```python
from build123d import *

# Parameters (mm, degrees)
BOSS_EXTRUDE1_DEPTH = 7.5
CHAMFER1_SIZE       = 2.5
SKETCH3_W           = 20
SKETCH3_H           = 20
BOSS_EXTRUDE2_DEPTH = 10
CHAMFER4_SIZE       = 2.5
SKETCH6_R           = 5
BOSS_EXTRUDE3_DEPTH = 10
CUT_EXTRUDE3_DEPTH  = 17
SKETCH11_R          = 30
SKETCH11_R_2        = 20
BOSS_EXTRUDE4_DEPTH = 20
CHAMFER5_SIZE2      = 20
CHAMFER5_SIZE       = 5
CHAMFER6_SIZE       = 2.5


with BuildPart() as part:
    # Sketch2 → Boss-Extrude1 (new, symmetric)
    with BuildSketch(Plane.XY):
        with BuildLine():
            ThreePointArc((84.922137279, 7.499595816), (1.268561005, 10.133701432), (-81.871756055, 19.753837344))
            ThreePointArc((-81.871756055, 19.753837344), (-104.803696773, 2.795280684), (-87.461525308, -19.847944306))
            ThreePointArc((-87.461525308, -19.847944306), (0.380210023, -22.09713345), (86.984359422, -7.232725467))
            ThreePointArc((86.984359422, -7.232725467), (92.427584063, 1.039709088), (84.922137279, 7.499595816))
        make_face()
    extrude(amount=BOSS_EXTRUDE1_DEPTH, both=True)

    # Chamfer1
    chamfer1_edges = [part.edges().sort_by_distance(p)[0] for p in [
        (92.427584063, 1.039709088, 7.5),
        (1.268561005, 10.133701432, 7.5),
        (-104.803696773, 2.795280684, 7.5),
        (0.380210023, -22.09713345, 7.5),
        (-104.803696773, 2.795280684, -7.5),
        (1.268561005, 10.133701432, -7.5),
        (92.427584063, 1.039709088, -7.5),
        (0.380210023, -22.09713345, -7.5),
    ]]
    chamfer(chamfer1_edges, length=CHAMFER1_SIZE)

    # Sketch3 → Boss-Extrude2 (add)
    with BuildSketch(Plane.XY.offset(7.5)):
        with Locations((-85, 0)):
            Rectangle(SKETCH3_W, SKETCH3_H)
    extrude(amount=BOSS_EXTRUDE2_DEPTH)

    # Chamfer4
    chamfer4_edges = [part.edges().sort_by_distance(p)[0] for p in [
        (-75, 0, 17.5),
        (-85, 10, 17.5),
        (-95, 0, 17.5),
        (-85, -10, 17.5),
    ]]
    chamfer(chamfer4_edges, length=CHAMFER4_SIZE)

    # Sketch6 → Boss-Extrude3 (add)
    with BuildSketch(Plane(origin=(0, 0, -7.5), x_dir=(-1, 0, 0), z_dir=(0, 0, -1))):
        with Locations(Location((85, 0, 0), (0, 0, 180))):
            Circle(SKETCH6_R)
    extrude(amount=BOSS_EXTRUDE3_DEPTH)

    # Sketch7 → Cut-Extrude3 (cut, symmetric)
    with BuildSketch(Plane(origin=(0, 0, 0), x_dir=(1, 0, 0), z_dir=(0, 1, 0))):
        with BuildLine():
            ThreePointArc((101.914257425, 20), (87.772121801, 14.142135624), (81.914257425, 0))
            Line((81.914257425, 0), (101.914257425, 0))
            Line((101.914257425, 0), (101.914257425, 20))
        make_face()
        with BuildLine():
            Line((101.914257425, 0), (81.914257425, 0))
            ThreePointArc((81.914257425, 0), (87.772121801, -14.142135624), (101.914257425, -20))
            Line((101.914257425, -20), (101.914257425, 0))
        make_face()
    extrude(amount=CUT_EXTRUDE3_DEPTH, both=True, mode=Mode.SUBTRACT)

    # Sketch7<5> one side → Revolve2 (revolve)
    with BuildSketch(Plane(origin=(0, 0, 0), x_dir=(1, 0, 0), z_dir=(0, 1, 0)), mode=Mode.PRIVATE) as revolve2_sk:
        with BuildLine():
            Line((101.914257425, 20), (101.914257425, 30))
            ThreePointArc((101.914257425, 30), (80.701053989, 21.213203436), (71.914257425, 0))
            Line((71.914257425, 0), (81.914257425, 0))
            ThreePointArc((81.914257425, 0), (87.772121801, 14.142135624), (101.914257425, 20))
        make_face()
    revolve(revolve2_sk.sketch.rotate(Axis((-136.30632513, 0, 0), (1, 0, 0)), 180), axis=Axis((-136.30632513, 0, 0), (1, 0, 0)))

    # Sketch11 → Boss-Extrude4 (add)
    with BuildSketch(Plane(origin=(101.914257425, 0, 0), x_dir=(0, 0, -1), z_dir=(1, 0, 0))):
        Circle(SKETCH11_R)
        with Locations(Location((0, 0, 0), (0, 0, 180))):
            Circle(SKETCH11_R_2, mode=Mode.SUBTRACT)
    extrude(amount=BOSS_EXTRUDE4_DEPTH)

    # Chamfer5
    chamfer5_edges = [part.edges().sort_by_distance(p)[0] for p in [
        (121.914257425, 0, -20),
    ]]
    chamfer5_side = [part.faces().sort_by_distance(p)[0] for p in [
        (121.914257425, 0, -20.1),
    ]]
    chamfer(chamfer5_edges, length=CHAMFER5_SIZE - 0.0001, length2=CHAMFER5_SIZE2 - 0.0001, reference=chamfer5_side[0])  # a hair under: the kernel refuses the full size

    # Chamfer6
    chamfer6_edges = [part.edges().sort_by_distance(p)[0] for p in [
        (121.914257425, 0, 30),
    ]]
    chamfer(chamfer6_edges, length=CHAMFER6_SIZE)


solid = part.part
```
Verification items for the finished model (mm, model axes). A direction names the side the tool comes from. Coordinates: 2 decimals unless noted, no trailing zeros. Write each loop counter-clockwise with the first axis right and the second up, starting at its lowest first coordinate (ties: lowest second). Pieces come first, ordered by that corner, then holes. Notation, with made-up numbers: (11.25, 18) - (31.25, 18) arc R16 ccw to (31.25, 26) - close; hole circle Ø4 at (79.25, 73). An arc over 180 degrees is marked (long way). One line per question, with ' | ' between items. Start each with the question number.
1. Access from +Z, -Z, +X, -X, +Y, -Y to the whole of each face (thin tool, end or side, straight path). Record for faces 1 (the flat face through (-85, 0, -17.5)), 2 (the flat face through (-85, 0, 17.5)), 3 (the flat face through (-75, 0, 11)), 4 (the cylindrical face through (-80.381, 1.915, -12.43)).
2. Section check B-B (x = 89). Enter the section's corners in (y, z), plus the area to 3 significant figures.
3. Gauge pin test, flat ends, axial feed: P1, Ø8, axis at x = 53, y = 8.5, coming from the -Z side; P2, Ø12, axis at x = -83.5, y = 3.5, coming from the +Z side; P3, Ø3, axis at x = -82.5, z = -7, coming from the +Y side. Record the tip position at first contact, or that the pin passes through.
4. Material ranges on line 1 along Y through (x, z) = (101, 0); line 2 along X through (y, z) = (0.5, 15.5); line 3 along Z through (x, y) = (52.5, -11.5), recorded low to high.
5. Draft check along Z on faces 5 (the flat face through (-35, -6, -7.5)), 6 (the flat face through (121.914, -22.3, -12.1)), 7 (the conical face through (107.33, -21.172, -2.78)), 8 (the conical face through (121.758, 8.307, -26.379)). Enter one of: released by +Z, released by -Z, zero draft, split by the parting line, or undercut.
Computed values:
1) face 1: -Z, -X, +Y, -Y | face 2: +Z, -X, +Y, -Y | face 3: +Z, +Y, -Y | face 4: -Z
2) outline: circle Ø54.16 at (0, 0); hole circle Ø30.54 at (0, 0) | area: 1,570 mm²
3) P1: z = -7.5 | P2: z = 17.5 | P3: y = 19.35
4) line 1: -29.99 to -19.98, 19.98 to 29.99 | line 2: -94.5 to -75.5, 76.23 to 89.28 | line 3: -7.5 to 7.5
5) face 5: released by -Z | face 6: zero draft | face 7: undercut | face 8: split by the parting line
